Verification items for this drawing (mm, ordinates from the low corner). A direction names the side the tool comes from. Round coordinates to 2 decimals unless told otherwise and drop trailing zeros. Order: outer loops, then holes, each group sorted by start corner. A loop starts at its lowest first (then second) coordinate and runs counter-clockwise, first axis right, second up.
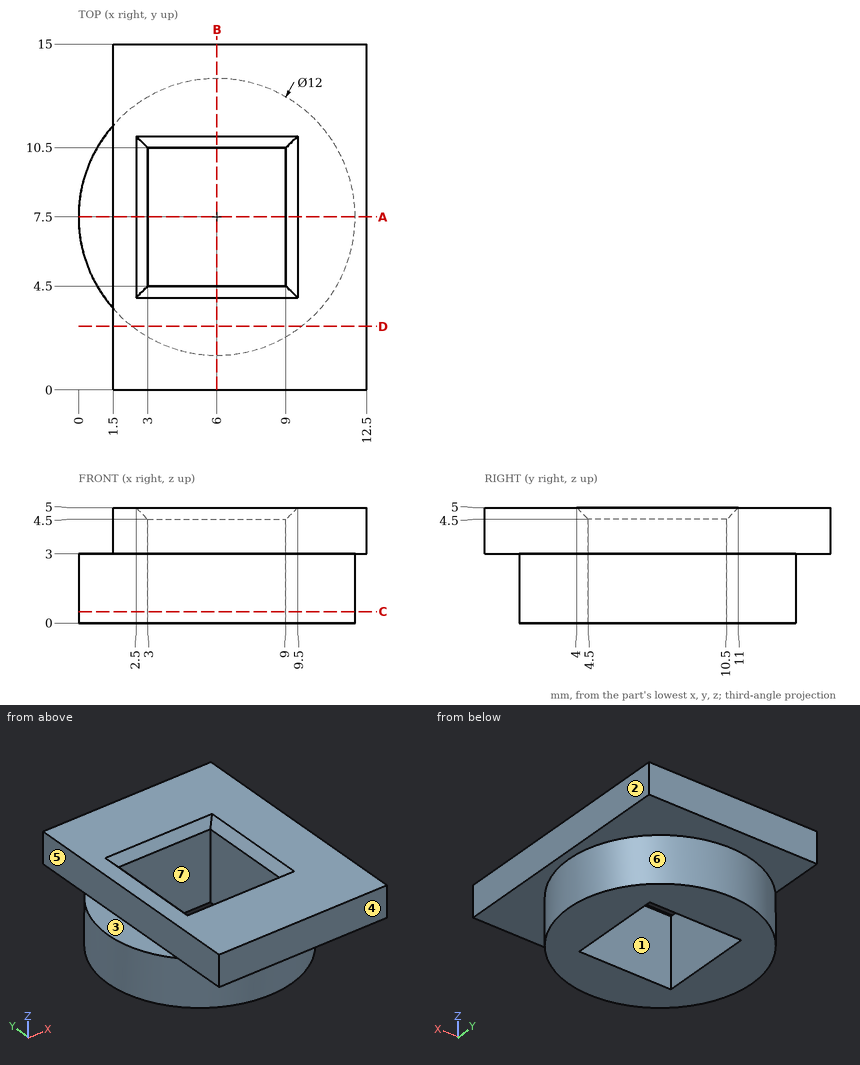
Item 1: Sectioned sample at C-C (z = 0.5). Record the cut outline in (x, y).
Answer:
outline: circle Ø12 at (6, 7.5); hole (3, 4.5) - (9, 4.5) - (9, 10.5) - (3, 10.5) - close
Item 2: Sectioned sample at B-B (x = 6). Record the cut outline in (y, z).
Answer:
outline: (0, 3) - (1.5, 3) - (1.5, 0) - (4.5, 0) - (4.5, 4.5) - (4, 5) - (0, 5) - close; (10.5, 0) - (13.5, 0) - (13.5, 3) - (15, 3) - (15, 5) - (11, 5) - (10.5, 4.5) - close
Item 3: Release check for a two-part mould opening along X. For the marked faces 1, 2 and 3 record: released by +X, released by -X, zero draft, split by the parting line, or undercut.
Answer:
face 1: undercut
face 2: released by +X
face 3: zero draft
Item 4: Access from +Z, -Z, +X, -X, +Y, -Y to the whole of each face (thin tool, end or side, straight path). Record for the marked faces 4, 5, 6 and 7.
Answer:
face 4: +Z, -Z, +X, -X, -Y
face 5: +Z, -X, +Y, -Y
face 6: -Z
face 7: +Z, -Z
Item 5: Scan lines: line 1 along X through (y, z) = (6.5, 3.15); line 2 along Z through (x, y) = (3.25, 13.25); line 3 along Y through (x, z) = (8, 4.3). Record each from-to range of solid material in increasing order.
Answer:
line 1: x = 1.5 to 3, 9 to 12.5
line 2: z = 3 to 5
line 3: y = 0 to 4.5, 10.5 to 15
Item 6: Go/stop test with flat-tipped pins: P1, Ø1.6, axis at y = 10, z = 4, coming from the -X side; P2, Ø0.8, axis at x = 1, y = 9, coming from the +Z side. Record where each tip stops, or that it passes through.
Answer:
P1: stops at x = 1.5
P2: stops at z = 3
Item 7: Sectioned sample at D-D (y = 2.75). Record the cut outline in (x, z), and give its area (3 significant figures).
Answer:
outline: (1.5, 3) - (2.33, 3) - (2.33, 0) - (9.67, 0) - (9.67, 3) - (12.5, 3) - (12.5, 5) - (1.5, 5) - close
area: 44.0 mm2
Item 8: Sectioned sample at A-A (y = 7.5). Record the cut outline in (x, z).
Answer:
outline: (0, 0) - (3, 0) - (3, 4.5) - (2.5, 5) - (1.5, 5) - (1.5, 3) - (0, 3) - close; (9, 0) - (12, 0) - (12, 3) - (12.5, 3) - (12.5, 5) - (9.5, 5) - (9, 4.5) - close
